from build123d import *

# Parameters (mm, degrees)
F1_DEPTH = 3
F2_R     = 2
F3_W     = 10.639583
F3_H     = 3
F4_DEPTH = 1
F5_SIZE  = 0.5


with BuildPart() as f1:
    # F0 (on Top) → F1 (new body)
    with BuildSketch(Plane.XY):
        with BuildLine():
            Line((-33.3, 41.75), (-33.3, -41.75))
            ThreePointArc((-33.3, -41.75), (-30.546804, -48.396804), (-23.9, -51.15))
            Line((-23.9, -51.15), (23.9, -51.15))
            ThreePointArc((23.9, -51.15), (30.546804, -48.396804), (33.3, -41.75))
            Line((33.3, -41.75), (33.3, 41.75))
            ThreePointArc((33.3, 41.75), (30.546804, 48.396804), (23.9, 51.15))
            Line((23.9, 51.15), (-23.9, 51.15))
            ThreePointArc((-23.9, 51.15), (-30.546804, 48.396804), (-33.3, 41.75))
        make_face()
        with BuildLine():
            ThreePointArc((27.3, -41.75), (26.304163, -44.154163), (23.9, -45.15))
            Line((23.9, -45.15), (-23.9, -45.15))
            ThreePointArc((-23.9, -45.15), (-26.304163, -44.154163), (-27.3, -41.75))
            Line((-27.3, -41.75), (-27.3, 41.75))
            ThreePointArc((-27.3, 41.75), (-26.304163, 44.154163), (-23.9, 45.15))
            Line((-23.9, 45.15), (23.9, 45.15))
            ThreePointArc((23.9, 45.15), (26.304163, 44.154163), (27.3, 41.75))
            Line((27.3, 41.75), (27.3, -41.75))
        make_face(mode=Mode.SUBTRACT)
    extrude(amount=F1_DEPTH)

    # F2
    f2_edges = [f1.edges().sort_by_distance(p)[0] for p in [
        (-33.3, 0, 3),
    ]]
    fillet(f2_edges, radius=F2_R)

    # F3 (on face) → F4 (join)
    with BuildSketch(Plane(origin=(0, 0, 0), x_dir=(1, 0, 0), z_dir=(0, 0, -1))):
        with Locations((-13.319791, -45.15)):
            Rectangle(F3_W, F3_H)
        with Locations((13.319791, -45.15)):
            Rectangle(F3_W, F3_H)
        with Locations((-13.319791, 45.15)):
            Rectangle(F3_W, F3_H)
        with Locations((13.319791, 45.15)):
            Rectangle(F3_W, F3_H)
    extrude(amount=F4_DEPTH)

    # F5
    f5_edges = [f1.edges().sort_by_distance(p)[0] for p in [
        (0, 45.15, 3),
        (-27.3, 0, 0),
        (-33.3, 0, 0),
    ]]
    chamfer(f5_edges, length=F5_SIZE)


solid = f1.part
Here's how the part is built. I have some questions about the finished solid (model axes, mm). A direction names the side the tool comes from. Round coordinates to 2 decimals unless told otherwise and drop trailing zeros. Write each loop counter-clockwise with the first axis right and the second up, starting at its lowest first coordinate (ties: lowest second). Pieces come first, ordered by that corner, then holes. Notation, with made-up numbers: (-38.5, 77) -> (12.5, 77) arc R22 cw to (12.5, 110) -> close; hole circle Ø7 at (42, 87.5). An arc over 180 degrees is marked (long way). One line per item, written item: value.
1) For faces 4 (the face through (-32.73, -0.58, 2.4)), 5 (the face through (-26.427, 44.222, 0.365)), 6 (the face through (-30.62, -48.32, 0.75)), 7 (the face through (26.28, 44.18, 1.23)), 8 (the face through (0, -45.15, 1)), which set-ups out of +Z, -Z, +X, -X, +Y, -Y let a thin tool reach every point of the face, with its end or its side?
Filled sheet:
face 4: +Z, -X, +Y, -Y
face 5: -Z
face 6: +Z, -Z, -X, -Y
face 7: +Z, -Z
face 8: +Z
2) Suppose I cut it at C-C on x = -6. List the corners of the cut face in (y, z) for me, plus the area to 3 significant figures.
Filled sheet:
outline: (-51.15, 0.5) -> (-50.65, 0) -> (-45.15, 0) -> (-45.15, 2.5) -> (-45.65, 3) -> (-49.15, 3) arc R2 ccw to (-51.15, 1) -> close; (45.15, 0) -> (50.65, 0) -> (51.15, 0.5) -> (51.15, 1) arc R2 ccw to (49.15, 3) -> (45.65, 3) -> (45.15, 2.5) -> close
area: 33.8 mm2
3) I'm going to push flat-ended pins straight in: pin 1 Ø0.8 at (y, z) = (44.5, -0.5) entering from +X; pin 2 Ø0.6 at (y, z) = (-16.5, 1.5) entering from +X; pin 3 Ø0.5 at (x, z) = (13.5, -0.5) entering from -Y. Where does each tip first touch, or does it pass through?
Filled sheet:
pin 1: stops at x = 18.64
pin 2: stops at x = 33.29
pin 3: stops at y = -46.65
4) If I drill on line 1 (Y direction, x = -7, z = 0.55); line 2 (X direction, y = 18.5, z = 1.3); line 3 (Y direction, x = -16, z = 1.3), over which ranges is the centre line in solid material (lowest first)? Write a range as [from, to].
Filled sheet:
line 1: y = [-51.15, -45.15], [45.15, 51.15]
line 2: x = [-33.28, -27.3], [27.3, 33.28]
line 3: y = [-51.13, -45.15], [45.15, 51.13]
5) Suppose I cut it at B-B on y = -12. List the corners of the cut face in (x, z) for me.
Filled sheet:
outline: (-33.3, 0.5) -> (-32.8, 0) -> (-27.8, 0) -> (-27.3, 0.5) -> (-27.3, 2.5) -> (-27.8, 3) -> (-31.3, 3) arc R2 ccw to (-33.3, 1) -> close; (27.3, 0) -> (32.8, 0) -> (33.3, 0.5) -> (33.3, 1) arc R2 ccw to (31.3, 3) -> (27.8, 3) -> (27.3, 2.5) -> close
6) We'd pull the mould along X, two halves only. Please class faces 1 (the face through (-30.22, 48.21, 0.14)), 2 (the face through (26.43, -44.23, 2.64)), 3 (the face through (0.33, -50.58, 2.4)): released by +X, released by -X, zero draft, split by the parting line, or undercut.
Filled sheet:
face 1: released by -X
face 2: undercut
face 3: zero draft
7) Suppose I cut it at A-A on x = -22. List the corners of the cut face in (y, z) for me, plus the area to 3 significant figures.
Filled sheet:
outline: (-51.15, 0.5) -> (-50.65, 0) -> (-45.65, 0) -> (-45.15, 0.5) -> (-45.15, 2.5) -> (-45.65, 3) -> (-49.15, 3) arc R2 ccw to (-51.15, 1) -> close; (45.15, 0.5) -> (45.65, 0) -> (50.65, 0) -> (51.15, 0.5) -> (51.15, 1) arc R2 ccw to (49.15, 3) -> (45.65, 3) -> (45.15, 2.5) -> close
area: 33.5 mm2
